```python
from build123d import *

# Parameters (mm, degrees)
SKETCH1_W                  = 38
SKETCH1_H                  = 12
BOSS_EXTRUDE1_DEPTH        = 1.2
SKETCH2_W                  = 29
SKETCH2_H                  = 11.5
BOSS_EXTRUDE2_DEPTH        = 1.5
BOSS_EXTRUDE3_START        = -9.8
SKETCH3_R                  = 0.25
BOSS_EXTRUDE3_DEPTH        = 11.4
CHAMFER1_SIZE              = 0.1
FILLET1_R                  = 0.5
LPATTERN1_COUNT            = 4
LPATTERN1_PITCH            = 2.54
CHAMFER1_OF_LPATTERN1_SIZE = 0.1
FILLET1_OF_LPATTERN1_R     = 0.5
SKETCH4_W                  = 2.5
SKETCH4_H                  = 10.5
BOSS_EXTRUDE4_DEPTH        = 2.5
FILLET2_R                  = 0.5
SKETCH5_W                  = 3
SKETCH5_H                  = 11.5
CUT_EXTRUDE1_DEPTH         = 0.15


with BuildPart() as part:
    # Sketch1 → Boss-Extrude1 (new body)
    with BuildSketch(Plane(origin=(0, 0, 0), x_dir=(1, 0, 0), z_dir=(0, 1, 0))):
        Rectangle(SKETCH1_W, SKETCH1_H)
    extrude(amount=BOSS_EXTRUDE1_DEPTH)

    # Sketch2 → Boss-Extrude2 (add)
    with BuildSketch(Plane(origin=(0, 1.2, 0), x_dir=(1, 0, 0), z_dir=(0, 1, 0))):
        with Locations((0.5, 0)):
            Rectangle(SKETCH2_W, SKETCH2_H)
    extrude(amount=BOSS_EXTRUDE2_DEPTH)

    # Sketch3 → Boss-Extrude3 (add)
    with BuildSketch(Plane(origin=(0, 1.2, 0), x_dir=(1, 0, 0), z_dir=(0, 1, 0)).offset(BOSS_EXTRUDE3_START)):
        with Locations((-17.35, -3.81)):
            Circle(SKETCH3_R)
    boss_extrude3 = extrude(amount=BOSS_EXTRUDE3_DEPTH)

    # Chamfer1
    chamfer1_edges = [part.edges().sort_by_distance(p)[0] for p in [
        (-17.6, 2.8, 3.81),
    ]]
    chamfer(chamfer1_edges, length=CHAMFER1_SIZE)

    # Fillet1
    fillet1_edges = [part.edges().sort_by_distance(p)[0] for p in [
        (-17.6, 1.2, 3.81),
    ]]
    fillet(fillet1_edges, radius=FILLET1_R)

    # LPattern1: Boss-Extrude3 ×4
    with Locations(*[(0, 0, -i * LPATTERN1_PITCH) for i in range(1, LPATTERN1_COUNT)]):
        add(boss_extrude3)

    # Chamfer1 of LPattern1
    chamfer1_of_lpattern1_edges = [part.edges().sort_by_distance(p)[0] for p in [
        (-17.6, 2.8, 1.27),
        (-17.6, 2.8, -1.27),
        (-17.6, 2.8, -3.81),
    ]]
    chamfer(chamfer1_of_lpattern1_edges, length=CHAMFER1_OF_LPATTERN1_SIZE)

    # Fillet1 of LPattern1
    fillet1_of_lpattern1_edges = [part.edges().sort_by_distance(p)[0] for p in [
        (-17.6, 1.2, 1.27),
        (-17.6, 1.2, -1.27),
        (-17.6, 1.2, -3.81),
    ]]
    fillet(fillet1_of_lpattern1_edges, radius=FILLET1_OF_LPATTERN1_R)

    # Sketch4 → Boss-Extrude4 (add)
    with BuildSketch(Plane.XZ):
        with Locations((-17.35, 0)):
            Rectangle(SKETCH4_W, SKETCH4_H)
    extrude(amount=BOSS_EXTRUDE4_DEPTH)

    # Fillet2
    fillet2_edges = [part.edges().sort_by_distance(p)[0] for p in [
        (-16.1, -1.25, -5.25),
        (-16.1, -1.25, 5.25),
        (-18.6, -1.25, 5.25),
        (-18.6, -1.25, -5.25),
    ]]
    fillet(fillet2_edges, radius=FILLET2_R)

    # Sketch5 → Cut-Extrude1 (cut)
    with BuildSketch(Plane(origin=(0, 2.7, 0), x_dir=(1, 0, 0), z_dir=(0, 1, 0))):
        with Locations((13.5, 0)):
            Rectangle(SKETCH5_W, SKETCH5_H)
    extrude(amount=-CUT_EXTRUDE1_DEPTH, mode=Mode.SUBTRACT)


solid = part.part
```
Build history of the part. All positions in model axes, mm. A direction names the side the tool comes from. Coordinates: 2 decimals unless noted, no trailing zeros. Order: outer loops, then holes, each group sorted by start corner. A loop starts at its lowest first (then second) coordinate and runs counter-clockwise, first axis right, second up.
Item 1: Saw through at B-B on x = 1.5. List the corners of the cut face in (y, z), then the cut area to 4 significant figures.
Filled in:
outline: (0, -6) - (1.2, -6) - (1.2, -5.75) - (2.7, -5.75) - (2.7, 5.75) - (1.2, 5.75) - (1.2, 6) - (0, 6) - close
area: 31.65 mm2
Item 2: Saw through at A-A on y = -3.25. List the corners of the cut face in (x, z), then the cut area to 3 significant figures.
Filled in:
outline: circle Ø0.5 at (-17.35, -3.81); circle Ø0.5 at (-17.35, -1.27); circle Ø0.5 at (-17.35, 1.27); circle Ø0.5 at (-17.35, 3.81)
area: 0.785 mm2
Item 3: Tool access for faces 4 (the flat face through (-17, -1, -5.25)), 5 (the flat face through (-1, 2.7, 0)), 6 (the flat face through (-18.6, -1, 0)): list every direction of +Z, -Z, +X, -X, +Y, -Y with a clear straight run to the whole face (end or side of a thin tool).
Filled in:
face 4: -Z, +X, -X, -Y
face 5: +Z, -Z, +X, +Y
face 6: +Z, -Z, -X, -Y
Item 4: Saw through at C-C on y = -1.25. List the corners of the cut face in (x, z), then the cut area to 3 significant figures.
Filled in:
outline: (-18.6, -4.75) arc R0.5 ccw to (-18.1, -5.25) - (-16.6, -5.25) arc R0.5 ccw to (-16.1, -4.75) - (-16.1, 4.75) arc R0.5 ccw to (-16.6, 5.25) - (-18.1, 5.25) arc R0.5 ccw to (-18.6, 4.75) - close
area: 26.0 mm2
Item 5: Drill centre lines: L1, parallel to X at y = 1.75, z = 3.75; L2, parallel to X at y = -0.25, z = -4; L3, parallel to Y at x = 10, z = 1. Where is each one in solid material? Low to high.
Filled in:
L1: x = -17.59 to -17.11, -14 to 15
L2: x = -18.6 to -16.1
L3: y = 0 to 2.7
Item 6: Mould opens along X. For faces 1 (the flat face through (-16.1, -1, 0)), 2 (the flat face through (-19, 1, 0)), 3 (the flat face through (-14, 2, 0)) say: released by +X, released by -X, zero draft, split by the parting line, or undercut.
Filled in:
face 1: released by +X
face 2: released by -X
face 3: undercut
Item 7: Drop flat-ended pins along their axis: pin 1 Ø3.5 at (x, z) = (-5, 0.5) entering from -Y; pin 2 Ø1.2 at (x, y) = (-17, -2) entering from -Z; pin 3 Ø0.9 at (x, z) = (14, -2.5) entering from +Y. Give the stop position or say it passes through.
Filled in:
pin 1: stops at y = 0
pin 2: stops at z = -5.25
pin 3: stops at y = 2.55
